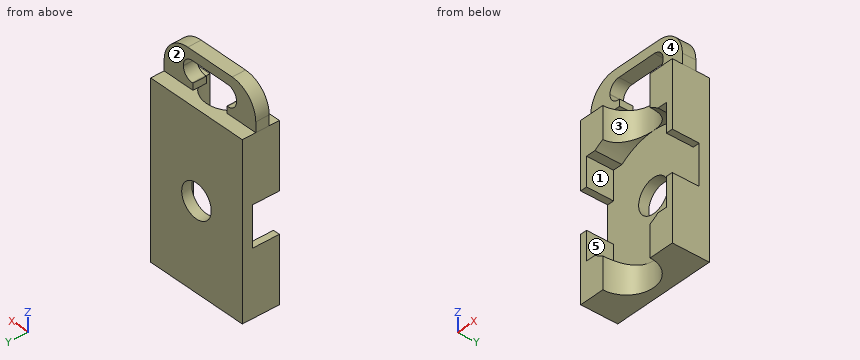
```python
from build123d import *

# Parameters (mm, degrees)
SKETCH_1_W               = 31
SKETCH_1_H               = 51
EXTRUDE_1_DEPTH          = 0.0001
EXTRUDE_1_DEPTH_BACK     = 11
SKETCH_2_W               = 27
SKETCH_2_H               = 12
SKETCH_2_R               = 5
SKETCH_2_W_2             = 2
CUT_EXTRUDE_1_DEPTH      = 0.0001
CUT_EXTRUDE_1_DEPTH_BACK = 8
SKETCH_3_R               = 5
CUT_EXTRUDE_3_DEPTH      = 12
SKETCH_4_R               = 8
CUT_EXTRUDE_4_DEPTH      = 102
EXTRUDE_2_DEPTH          = 4


with BuildPart() as part:
    # Эскиз1 → Бобышка-Вытянуть1 (new, two sides)
    with BuildSketch(Plane(origin=(0, 0, 0), x_dir=(1, 0, 0), z_dir=(0, 1, 0))) as extrude_1_sk:
        Rectangle(SKETCH_1_W, SKETCH_1_H)
    extrude(amount=EXTRUDE_1_DEPTH)
    extrude(extrude_1_sk.sketch, amount=-EXTRUDE_1_DEPTH_BACK)

    # Эскиз2 → Вырез-Вытянуть1 (cut, two sides)
    with BuildSketch(Plane.XZ.offset(11)) as cut_extrude_1_sk:
        with BuildLine():
            Line((-13.5, 11.9058809), (-13.5, 6))
            Line((-13.5, 6), (13.5, 6))
            Line((13.5, 6), (13.5, 11.9058809))
            ThreePointArc((13.5, 11.9058809), (12.152101624, 13.27879611), (10.665364504, 14.5))
            Line((10.665364504, 14.5), (-10.665364504, 14.5))
            ThreePointArc((-10.665364504, 14.5), (-12.152101624, 13.27879611), (-13.5, 11.9058809))
        make_face()
        Rectangle(SKETCH_2_W, SKETCH_2_H)
        with Locations(Location((0, 0, 0), (0, 0, 90))):
            Circle(SKETCH_2_R, mode=Mode.SUBTRACT)
        with Locations((-14.5, 0)):
            Rectangle(SKETCH_2_W_2, SKETCH_2_H)
        with Locations((14.5, 0)):
            Rectangle(SKETCH_2_W_2, SKETCH_2_H)
        with BuildLine():
            Line((13.5, -6), (-13.5, -6))
            Line((-13.5, -6), (-13.5, -11.9058809))
            ThreePointArc((-13.5, -11.9058809), (-12.152101624, -13.27879611), (-10.665364504, -14.5))
            Line((-10.665364504, -14.5), (10.665364504, -14.5))
            ThreePointArc((10.665364504, -14.5), (12.152101624, -13.27879611), (13.5, -11.9058809))
            Line((13.5, -11.9058809), (13.5, -6))
        make_face()
        with BuildLine():
            Line((13.5, -14.5), (13.5, -11.9058809))
            ThreePointArc((13.5, -11.9058809), (12.152101624, -13.27879611), (10.665364504, -14.5))
            Line((10.665364504, -14.5), (13.5, -14.5))
        make_face()
        with BuildLine():
            Line((10.665364504, -14.5), (-10.665364504, -14.5))
            ThreePointArc((-10.665364504, -14.5), (0, -18), (10.665364504, -14.5))
        make_face()
        with BuildLine():
            ThreePointArc((-10.665364504, -14.5), (-12.152101624, -13.27879611), (-13.5, -11.9058809))
            Line((-13.5, -11.9058809), (-13.5, -14.5))
            Line((-13.5, -14.5), (-10.665364504, -14.5))
        make_face()
        with BuildLine():
            Line((-13.5, 14.5), (-13.5, 11.9058809))
            ThreePointArc((-13.5, 11.9058809), (-12.152101624, 13.27879611), (-10.665364504, 14.5))
            Line((-10.665364504, 14.5), (-13.5, 14.5))
        make_face()
        with BuildLine():
            ThreePointArc((10.665364504, 14.5), (0, 18), (-10.665364504, 14.5))
            Line((-10.665364504, 14.5), (10.665364504, 14.5))
        make_face()
        with BuildLine():
            ThreePointArc((10.665364504, 14.5), (12.152101624, 13.27879611), (13.5, 11.9058809))
            Line((13.5, 11.9058809), (13.5, 14.5))
            Line((13.5, 14.5), (10.665364504, 14.5))
        make_face()
    extrude(amount=CUT_EXTRUDE_1_DEPTH, mode=Mode.SUBTRACT)
    extrude(cut_extrude_1_sk.sketch, amount=-CUT_EXTRUDE_1_DEPTH_BACK, mode=Mode.SUBTRACT)

    # Эскиз3 → Вырез-Вытянуть3 (cut)
    with BuildSketch(Plane.XZ.offset(11)):
        with Locations(Location((0, 0, 0), (0, 0, 270))):
            Circle(SKETCH_3_R)
    extrude(amount=-CUT_EXTRUDE_3_DEPTH, mode=Mode.SUBTRACT)

    # Эскиз4 → Вырез-Вытянуть4 (cut)
    with BuildSketch(Plane.XY.offset(25.5)):
        with Locations((0, -11)):
            Circle(SKETCH_4_R)
    extrude(amount=-CUT_EXTRUDE_4_DEPTH, mode=Mode.SUBTRACT)

    # Sketch 1 2 → Бобышка-Вытянуть2 (add)
    with BuildSketch(Plane(origin=(-15.5, -3.9999, 25.5), x_dir=(0.9953500135553002, 0, 0.0963241948601902), z_dir=(0, -1, 0))):
        with BuildLine():
            Line((0, 0), (9.704662632, -0.9391609))
            Line((9.704662632, -0.9391609), (9.897311022, 1.051539127))
            Line((9.897311022, 1.051539127), (9.649856542, 1.075486335))
            ThreePointArc((9.649856542, 1.075486335), (7.62303842, 2.154414617), (6.952779086, 4.35050896))
            Line((6.952779086, 4.35050896), (6.964859124, 4.475336021))
            ThreePointArc((6.964859124, 4.475336021), (8.043787406, 6.502154143), (10.239881749, 7.172413477))
            Line((10.239881749, 7.172413477), (22.181315865, 6.01679082))
            ThreePointArc((22.181315865, 6.01679082), (24.208133987, 4.937862538), (24.878393321, 2.741768195))
            Line((24.878393321, 2.741768195), (24.866313283, 2.616941135))
            ThreePointArc((24.866313283, 2.616941135), (23.787385001, 0.590123012), (21.591290658, -0.080136321))
            Line((21.591290658, -0.080136321), (21.343836178, -0.056189114))
            Line((21.343836178, -0.056189114), (21.151187788, -2.046889141))
            Line((21.151187788, -2.046889141), (30.85585042, -2.986050041))
            Line((30.85585042, -2.986050041), (31.144823005, 0))
            ThreePointArc((31.144823005, 0), (29.357464781, 5.856251582), (23.952616455, 8.733393667))
            Line((23.952616455, 8.733393667), (9.022366252, 10.17825659))
            ThreePointArc((9.022366252, 10.17825659), (3.16611467, 8.390898367), (0.288972585, 2.986050041))
            Line((0.288972585, 2.986050041), (0, 0))
        make_face()
    extrude(amount=EXTRUDE_2_DEPTH)


solid = part.part
```
CAD build for the part. Positions are in the model's coordinates, mm. Face numbers are marked on the shaded views. A direction names the side the tool comes from. Coordinates: 2 decimals unless noted, no trailing zeros. Loops run counter-clockwise (first coordinate to the right, second up) from the corner with the lowest first, then second, coordinate; pieces in that order, holes last. Notation, with made-up numbers: (-25.75, 11.5) - (-18.75, 11.5) arc R24 ccw to (-18.75, 38.5) - close; hole circle Ø1 at (39.5, -8). An arc over 180 degrees is marked (long way). Use CSV: the item, a comma, the result in double quotes. Start each with the question number.
Q1. Drop flat-ended pins along their axis: P1, Ø5, axis at y = -10, z = 28.5, coming from the +X side; P2, Ø2, axis at x = -1.5, y = -7.5, coming from the -Z side; P3, Ø5, axis at x = 7, y = -1, coming from the +Z side; P4, Ø3.5, axis at x = 6.5, z = 33, coming from the -Y side. Give the stop position or say it passes through.
Q2. 3-axis set-ups, long thin cutter, end or side, ignore diameter. For the marked faces 3, 4 and 5: which of +Z, -Z, +X, -X, +Y, -Y reach the whole face in a straight line?
Q3. Probe probe 1 along X at (y, z) = (-10.5, -10.5); probe 2 along Z at (x, y) = (0, -0.85); probe 3 along Z at (x, y) = (8, -8.5). List the from-to ranges inside material, lowest first. Write a range as from..to.
Q4. Cut at D-D, the plane z = -21. List the corners of the cut face in (x, y), then the cut area to 3 significant figures.
Q5. Cut at C-C, the plane x = -3. List the corners of the cut face in (y, z), then the cut area to 3 significant figures.
Q6. Cut at B-B, the plane z = 0. List the corners of the cut face in (x, y).
Q7. Cut at A-A, the plane y = -1.25. List the corners of the cut face in (x, z).
Q8. Two-plate mould, pull along X, no slides. Class the marked faces 1 and 2: +X half, -X half, draft (parallel to the pull), parting line (faces both ways), or undercut.
Here are the results:
1,P1,"x = 15.5"
1,P2,"z = 33.63"
1,P3,"z = 25.5"
1,P4,"y = -8"
2,face 3,"-Z, -Y"
2,face 4,"+Z, +X, -X, -Y"
2,face 5,"-Y"
3,probe 1,"-15.5..-13.5, 13.5..15.5"
3,probe 2,"-25.5..-5, 5..25.5"
3,probe 3,"-25.5..-16.12, 16.12..25.5"
4,outline,"(-15.5, -11) - (-8, -11) arc R8 cw to (8, -11) - (15.5, -11) - (15.5, 0) - (-15.5, 0) - close"
4,area,"240 mm2"
5,outline,"(-8, 33.63) - (-4, 33.63) - (-4, 36.5) - (-8, 36.5) - close; (-3.58, -25.5) - (0, -25.5) - (0, -4) - (-3, -4) - (-3, -17.75) - (-3.58, -17.75) - close; (-3.58, 17.75) - (-3, 17.75) - (-3, 4) - (0, 4) - (0, 25.5) - (-3.58, 25.5) - close"
5,area,"150 mm2"
6,outline,"(-15.5, -3) - (-5, -3) - (-5, 0) - (-15.5, 0) - close; (5, -3) - (15.5, -3) - (15.5, 0) - (5, 0) - close"
7,outline,"(-15.5, -25.5) - (15.5, -25.5) - (15.5, 25.5) - (-15.5, 25.5) - close; hole circle Ø10 at (0, 0)"
8,face 1,"undercut"
8,face 2,"draft"
